from build123d import *
from build123d.topology import SkipClean

# Parameters (mm, degrees)
SKETCH_1_W           = 85
SKETCH_1_H           = 15
EXTRUDE_1_DEPTH      = 30
SKETCH_2_R           = 1.4
CUT_EXTRUDE_1_DEPTH  = 40
CUT_EXTRUDE_2_DEPTH  = 40
FILLET_1_R           = 4
SKETCH_5_R           = 1.8
CUT_EXTRUDE_3_DEPTH  = 5
CHAMFER_1_SIZE       = 0.5
CUT_EXTRUDE_4_DEPTH  = 24
FILLET_3_R           = 4
CUT_EXTRUDE_START    = -5
SKETCH_9_R           = 1.8
CUT_EXTRUDE_5_DEPTH  = 5
FILLET_4_R           = 2
EXTRUDE_3_DEPTH      = 1
EXTRUDE_3_DEPTH_BACK = 16
SKETCH_10_R          = 1.4
FILLET_START         = -8.5
FILLET_5_DEPTH       = 17


with BuildPart() as part:
    # 草图1 → 凸台-拉伸1 (new body)
    with BuildSketch(Plane(origin=(0, 0, 0), x_dir=(1, 0, 0), z_dir=(0, 1, 0))):
        Rectangle(SKETCH_1_W, SKETCH_1_H)
    extrude(amount=EXTRUDE_1_DEPTH)

    # 草图2 → 切除-拉伸1 (cut)
    with BuildSketch(Plane.XY.offset(7.5)):
        with Locations((-35, 24)):
            Circle(SKETCH_2_R)
        with Locations((35, 24)):
            Circle(SKETCH_2_R)
        with Locations((28, 4.255699158)):
            Circle(SKETCH_2_R)
        with Locations((-28, 4.255699158)):
            Circle(SKETCH_2_R)
    extrude(amount=-CUT_EXTRUDE_1_DEPTH, mode=Mode.SUBTRACT)

    # 草图3 → 切除-拉伸2 (cut)
    with BuildSketch(Plane.XY.offset(7.5)):
        Polygon((-27, 24), (27, 24), (21, 4.255699158), (-21, 4.255699158), align=None)
    extrude(amount=-CUT_EXTRUDE_2_DEPTH, mode=Mode.SUBTRACT)

    # 圆角1
    fillet_1_edges = [part.edges().sort_by_distance(p)[0] for p in [
        (-21, 4.255699158, 0),
        (-27, 24, 0),
        (27, 24, 0),
        (21, 4.255699158, 0),
    ]]
    fillet(fillet_1_edges, radius=FILLET_1_R)

    # 草图5 → 切除-拉伸3 (cut)
    with BuildSketch(Plane(origin=(0, 30, 0), x_dir=(1, 0, 0), z_dir=(0, 1, 0))):
        with Locations(Location((-35, 4.5, 0), (0, 0, 270))):
            Circle(SKETCH_5_R)
        with Locations(Location((35, 4.5, 0), (0, 0, 270))):
            Circle(SKETCH_5_R)
        with Locations(Location((-20, -4.5, 0), (0, 0, 270))):
            Circle(SKETCH_5_R)
        with Locations(Location((20, -4.5, 0), (0, 0, 270))):
            Circle(SKETCH_5_R)
    extrude(amount=-CUT_EXTRUDE_3_DEPTH, mode=Mode.SUBTRACT)

    # 倒角1
    chamfer_1_edges = [part.edges().sort_by_distance(p)[0] for p in [
        (-42.5, 30, 0),
        (42.5, 30, 0),
        (-42.5, 0, 0),
        (42.5, 0, 0),
    ]]
    chamfer(chamfer_1_edges, length=CHAMFER_1_SIZE)

    # 草图6 → 切除-拉伸4 (cut)
    with BuildSketch(Plane.XY.offset(7.5)):
        Polygon((-42.5, 24), (-39.5, 24), (-33.5, 4.255699158), (-42.5, 4.255699158), align=None)
        Polygon((42.5, 24), (42.5, 4.255699158), (33.5, 4.255699158), (39.5, 24), align=None)
    extrude(amount=-CUT_EXTRUDE_4_DEPTH, mode=Mode.SUBTRACT)

    # 圆角3
    fillet_3_edges = [part.edges().sort_by_distance(p)[0] for p in [
        (-39.5, 24, 0),
        (39.5, 24, 0),
    ]]
    fillet(fillet_3_edges, radius=FILLET_3_R)

    # 草图9 → 切除-拉伸5 (cut)
    with BuildSketch(Plane.XZ.offset(CUT_EXTRUDE_START)):
        with Locations(Location((20, 4.5, 0), (0, 0, 90))):
            Circle(SKETCH_9_R)
        with Locations(Location((-20, 4.5, 0), (0, 0, 90))):
            Circle(SKETCH_9_R)
        with Locations(Location((-35, -4.5, 0), (0, 0, 90))):
            Circle(SKETCH_9_R)
        with Locations(Location((35, -4.5, 0), (0, 0, 90))):
            Circle(SKETCH_9_R)
    extrude(amount=CUT_EXTRUDE_5_DEPTH, mode=Mode.SUBTRACT)

    # 圆角4
    # the kernel refuses this fillet: 2 mm, written as the material it adds along each edge
    with BuildSketch(Plane(origin=(-33.5, 4.255699158, 7.5), x_dir=(-1, 0, 0), z_dir=(0, 0, -1))) as fillet_4_piece_1_section:
        with BuildLine():
            CenterArc((FILLET_4_R * 1.34903882702, FILLET_4_R), FILLET_4_R, 163.096751643, 106.903248357)
            Line((FILLET_4_R * 0.392241725729, FILLET_4_R * 1.29075643923), (0, 0))
            Line((0, 0), (FILLET_4_R * 1.34903882702, 0))
        make_face()
    fillet_4_piece_1 = extrude(amount=17.750206698, mode=Mode.PRIVATE)
    fillet_4_piece_1 = split(fillet_4_piece_1, bisect_by=Plane(origin=(-33.5, 4.255699158, -7.5), z_dir=(0, 0, 1)), keep=Keep.TOP, mode=Mode.PRIVATE)
    fillet_4_piece_1 = fillet_4_piece_1 - Plane(origin=(-35, 4.255699158, -4.5), x_dir=(0, 0, 1), z_dir=(0, 1, 0)) * Cylinder(1.8, 47, mode=Mode.PRIVATE)
    add(fillet_4_piece_1)
    with BuildSketch(Plane(origin=(-33.5, 4.255699158, 7.5), x_dir=(-1, 0, 0), z_dir=(0, 0, -1))) as fillet_4_piece_2_section:
        with BuildLine():
            CenterArc((FILLET_4_R * 1.34903882702, FILLET_4_R), FILLET_4_R, 163.096751643, 106.903248357)
            Line((FILLET_4_R * 0.392241725729, FILLET_4_R * 1.29075643923), (0, 0))
            Line((0, 0), (FILLET_4_R * 1.34903882702, 0))
        make_face()
    fillet_4_piece_2 = extrude(amount=17.750206698, mode=Mode.PRIVATE)
    fillet_4_piece_2 = split(fillet_4_piece_2, bisect_by=Plane(origin=(-33.5, 4.255699158, -7.5), z_dir=(0, 0, 1)), keep=Keep.TOP, mode=Mode.PRIVATE)
    fillet_4_piece_2 = split(fillet_4_piece_2, bisect_by=Plane(origin=(-33.5, 5, 7.5), z_dir=(0, 1, 0)), keep=Keep.TOP, mode=Mode.PRIVATE)
    add(fillet_4_piece_2)
    with BuildSketch(Plane(origin=(33.5, 4.255699158, 7.5), x_dir=(0.2907564392301515, 0.9567971012948373, 0), z_dir=(0, 0, -1))) as fillet_4_piece_3_section:
        with BuildLine():
            CenterArc((FILLET_4_R * 1.34903882702, FILLET_4_R), FILLET_4_R, 163.096751643, 106.903248357)
            Line((FILLET_4_R * 0.392241725729, FILLET_4_R * 1.29075643923), (0, 0))
            Line((0, 0), (FILLET_4_R * 1.34903882702, 0))
        make_face()
    fillet_4_piece_3 = extrude(amount=17.750206698, mode=Mode.PRIVATE)
    fillet_4_piece_3 = split(fillet_4_piece_3, bisect_by=Plane(origin=(33.5, 4.255699158, -7.5), z_dir=(0, 0, 1)), keep=Keep.TOP, mode=Mode.PRIVATE)
    fillet_4_piece_3 = fillet_4_piece_3 - Plane(origin=(35, 4.255699158, -4.5), x_dir=(0, 0, 1), z_dir=(0, 1, 0)) * Cylinder(1.8, 47, mode=Mode.PRIVATE)
    add(fillet_4_piece_3)
    with BuildSketch(Plane(origin=(33.5, 4.255699158, 7.5), x_dir=(0.2907564392301515, 0.9567971012948373, 0), z_dir=(0, 0, -1))) as fillet_4_piece_4_section:
        with BuildLine():
            CenterArc((FILLET_4_R * 1.34903882702, FILLET_4_R), FILLET_4_R, 163.096751643, 106.903248357)
            Line((FILLET_4_R * 0.392241725729, FILLET_4_R * 1.29075643923), (0, 0))
            Line((0, 0), (FILLET_4_R * 1.34903882702, 0))
        make_face()
    fillet_4_piece_4 = extrude(amount=17.750206698, mode=Mode.PRIVATE)
    fillet_4_piece_4 = split(fillet_4_piece_4, bisect_by=Plane(origin=(33.5, 4.255699158, -7.5), z_dir=(0, 0, 1)), keep=Keep.TOP, mode=Mode.PRIVATE)
    fillet_4_piece_4 = split(fillet_4_piece_4, bisect_by=Plane(origin=(33.5, 5, 7.5), z_dir=(0, 1, 0)), keep=Keep.TOP, mode=Mode.PRIVATE)
    add(fillet_4_piece_4)

    # 草图10 → 凸台-拉伸3 (add, two sides: drawn at the far end of the back side and taken through both)
    with SkipClean():  # the faces are left unmerged after this step: merging them gives an invalid solid
        with BuildSketch(Plane(origin=(0, 0, -7.5), x_dir=(-1, 0, 0), z_dir=(0, 0, -1)).offset(-EXTRUDE_3_DEPTH_BACK)):
            with BuildLine():
                Line((42.5, 29.5), (42, 30))
                Line((42, 30), (-42, 30))
                Line((-42, 30), (-42.5, 29.5))
                Line((-42.5, 29.5), (-42.5, 24))
                Line((-42.5, 24), (-39.5, 24))
                Line((-39.5, 24), (-38.637885631, 21.163025757))
                Line((-38.637885631, 21.163025757), (-34.284483451, 6.837212037))
                ThreePointArc((-34.284483451, 6.837212037), (-34.591368944, 5.064696589), (-36.198077654, 4.255699158))
                Line((-36.198077654, 4.255699158), (-42.5, 4.255699158))
                Line((-42.5, 4.255699158), (-42.5, 0.5))
                Line((-42.5, 0.5), (-42, 0))
                Line((-42, 0), (42, 0))
                Line((42, 0), (42.5, 0.5))
                Line((42.5, 0.5), (42.5, 4.255699158))
                Line((42.5, 4.255699158), (36.198077654, 4.255699158))
                ThreePointArc((36.198077654, 4.255699158), (34.591368944, 5.064696589), (34.284483451, 6.837212037))
                Line((34.284483451, 6.837212037), (38.637885631, 21.163025757))
                Line((38.637885631, 21.163025757), (39.5, 24))
                Line((39.5, 24), (42.5, 24))
                Line((42.5, 24), (42.5, 29.5))
            make_face()
            with Locations((-28, 4.255699158)):
                Circle(SKETCH_10_R, mode=Mode.SUBTRACT)
            with Locations((28, 4.255699158)):
                Circle(SKETCH_10_R, mode=Mode.SUBTRACT)
            with BuildLine():
                Line((-21.603844692, 24), (21.603844692, 24))
                ThreePointArc((21.603844692, 24), (24.817262112, 22.38200514), (25.431033097, 18.836974243))
                Line((25.431033097, 18.836974243), (21.862114369, 7.092673402))
                ThreePointArc((21.862114369, 7.092673402), (20.416931104, 5.042281739), (18.034925964, 4.255699158))
                Line((18.034925964, 4.255699158), (-18.034925964, 4.255699158))
                ThreePointArc((-18.034925964, 4.255699158), (-20.416931104, 5.042281739), (-21.862114369, 7.092673402))
                Line((-21.862114369, 7.092673402), (-25.431033097, 18.836974243))
                ThreePointArc((-25.431033097, 18.836974243), (-24.817262112, 22.38200514), (-21.603844692, 24))
            make_face(mode=Mode.SUBTRACT)
            with Locations((-35, 24)):
                Circle(SKETCH_10_R, mode=Mode.SUBTRACT)
            with Locations((35, 24)):
                Circle(SKETCH_10_R, mode=Mode.SUBTRACT)
        extrude(amount=EXTRUDE_3_DEPTH + EXTRUDE_3_DEPTH_BACK)
    add(part.part.scale(1), mode=Mode.REPLACE)  # the faces are merged on a copy

    # 圆角5: read off the stored shape, not the designer's step
    # 圆角5 outline → 圆角5 (add)
    with BuildSketch(Plane.XY.offset(FILLET_START)):
        with BuildLine():
            ThreePointArc((-42.465074036, 24), (-40.083068896, 23.21341742), (-38.637885631, 21.163025757))
            Line((-38.637885631, 21.163025757), (-39.5, 24))
            Line((-39.5, 24), (-42.465074036, 24))
        make_face()
        with BuildLine():
            ThreePointArc((38.637885631, 21.163025757), (40.083068896, 23.21341742), (42.465074036, 24))
            Line((42.465074036, 24), (39.5, 24))
            Line((39.5, 24), (38.637885631, 21.163025757))
        make_face()
    extrude(amount=FILLET_5_DEPTH)


solid = part.part
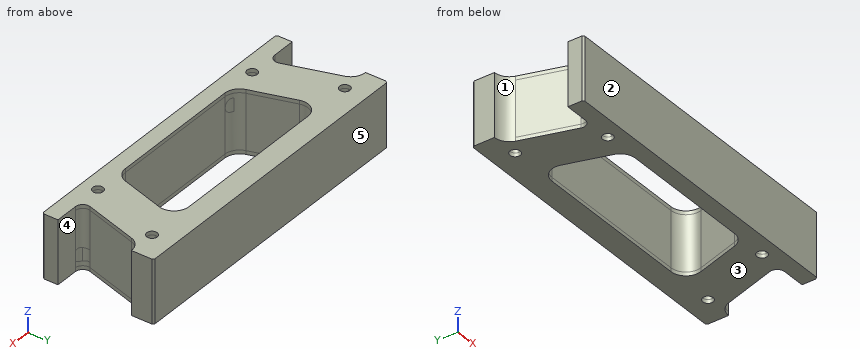
Work out the finished part from the listing and answer in its coordinate system (mm). Face numbers are marked on the shaded views. A direction names the side the tool comes from. Coordinates: 2 decimals unless noted, no trailing zeros. Order: outer loops, then holes, each group sorted by start corner. A loop starts at its lowest first (then second) coordinate and runs counter-clockwise, first axis right, second up. Notation, with made-up numbers: (20, 69.5) - (68, 69.5) arc R13 cw to (68, 86.5) - close; hole circle Ø9 at (74, 33). An arc over 180 degrees is marked (long way). Put each result on its own line as item: value. Start each with the question number.
1) Find section B-B (z = -4). State how many separate pieces and enclosed holes the cut face has, plus the area to 3 significant figures.
2) Find section A-A (x = 7.5). Give the vertices of the cut face in (y, z).
3) For a pull along Y with two mould halves and no side action, classify the marked faces 1, 2 and 3 as released by +Y, released by -Y, zero draft, split by the parting line, or undercut.
4) For the marked faces 4 and 5, determine the directions among +Z, -Z, +X, -X, +Y, -Y from which every point of the face is accessible in a straight line to the end or side of a thin tool.
5) Find section C-C (x = 28). Give the vertices of the cut face in (y, z), plus the area to 3 significant figures.
6) Flat-ended cylindrical pins translate along their axes: pin 1 (0.8 mm diameter, centred on x = 4.5, z = 8, fed in from -Y); pin 2 (5 mm diameter, centred on y = 8, z = 0, fed in from -X). Find the tip coordinate at first contact, or state that the pin passes through.
7) Find the intervals of material crossed by line 1 (Y direction, x = -28, z = -7.65); line 2 (Y direction, x = -4, z = -6.25); line 3 (X direction, y = 24.75, z = -4.5), in increasing order. Write a range as from..to.
Results list:
1. separate pieces: 1
1. enclosed holes: 5
1. area: 1,360 mm^2
2. outline: (0, -8.5) - (4.26, -8.5) - (4.26, 8.5) - (0, 8.5) - close; (24, -8.5) - (30, -8.5) - (30, 8.5) - (24, 8.5) - close
3. face 1: undercut
3. face 2: released by -Y
3. face 3: zero draft
4. face 4: +Z, -Z, +X
4. face 5: +Z, -Z, +X, -X, +Y
5. outline: (0, -8.5) - (2.86, -8.5) - (2.86, 8.5) - (0, 8.5) - close; (5.66, -8.5) - (30, -8.5) - (30, 8.5) - (5.66, 8.5) - close
5. area: 462 mm^2
6. pin 1: stops at y = 0
6. pin 2: stops at x = -35.4
7. line 1: y = 0..2.86, 5.66..30
7. line 2: y = 0..4.26, 24..30
7. line 3: x = -42.5..-36.18, -33.82..33.82, 36.18..42.5
